Geometry check sheet. Reference: the model listing, model coordinates, mm. Round coordinates to 2 decimals unless told otherwise and drop trailing zeros. Use one line per item in the form item = value.
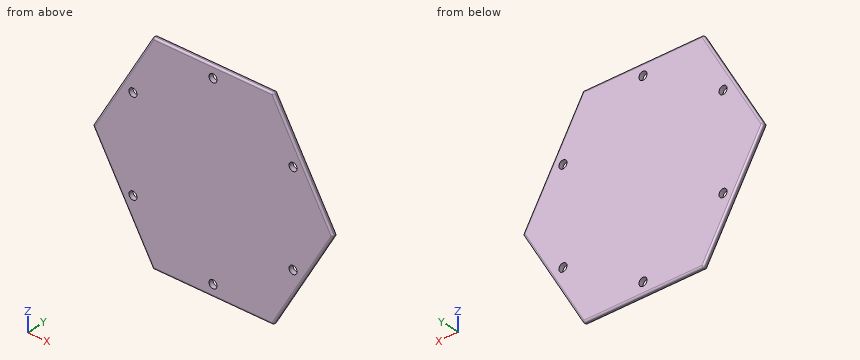
from build123d import *

# Parameters (mm, degrees)
BOSS_EXTRUDE1_DEPTH     = 2
FILLET3_R               = 0.75
CUT_EXTRUDE2_DEPTH      = 69.680097177
CUT_EXTRUDE2_DEPTH_BACK = 35
SKETCH3_R               = 1.75


with BuildPart() as part:
    # Sketch2 → Boss-Extrude1 (new body)
    with BuildSketch(Plane(origin=(0, 0, 0), x_dir=(1, 0, 0), z_dir=(0, 1, 0))):
        Polygon((51.961524227, 0), (25.980762114, 45), (-25.980762114, 45), (-51.961524227, 0), (-25.980762114, -45), (25.980762114, -45), align=None)
    extrude(amount=BOSS_EXTRUDE1_DEPTH)

    # Fillet3
    fillet3_edges = [part.edges().sort_by_distance(p)[0] for p in [
        (25.980762114, 1, 45),
        (-25.980762114, 1, 45),
        (-51.961524227, 1, 0),
        (-25.980762114, 1, -45),
        (25.980762114, 1, -45),
        (51.961524227, 1, 0),
        (0, 2, -45),
        (-38.97114317, 2, -22.5),
        (-38.97114317, 2, 22.5),
        (0, 2, 45),
        (38.97114317, 2, 22.5),
        (0, 0, 45),
        (-38.97114317, 0, 22.5),
        (-38.97114317, 0, -22.5),
        (0, 0, -45),
        (38.97114317, 0, -22.5),
        (38.97114317, 0, 22.5),
        (38.97114317, 2, -22.5),
    ]]
    fillet(fillet3_edges, radius=FILLET3_R)

    # Sketch3 → Cut-Extrude2 (cut, two sides: drawn at the far end of the back side and taken through both)
    with BuildSketch(Plane(origin=(0, 0, 0), x_dir=(1, 0, 0), z_dir=(0, 1, 0)).offset(-CUT_EXTRUDE2_DEPTH_BACK)):
        with Locations(Location((0, 40, 0), (0, 0, 270))):
            Circle(SKETCH3_R)
        with Locations(Location((34.641016151, 20, 0), (0, 0, 270))):
            Circle(SKETCH3_R)
        with Locations(Location((34.641016151, -20, 0), (0, 0, 270))):
            Circle(SKETCH3_R)
        with Locations(Location((0, -40, 0), (0, 0, 270))):
            Circle(SKETCH3_R)
        with Locations(Location((-34.641016151, -20, 0), (0, 0, 270))):
            Circle(SKETCH3_R)
        with Locations(Location((-34.641016151, 20, 0), (0, 0, 270))):
            Circle(SKETCH3_R)
    extrude(amount=CUT_EXTRUDE2_DEPTH + CUT_EXTRUDE2_DEPTH_BACK, mode=Mode.SUBTRACT)


solid = part.part
1. Material ranges on line 1 along Z through (x, y) = (0, 0.9); line 2 along X through (y, z) = (1.55, 20); line 3 along Z through (x, y) = (1.5, 0.35), recorded low to high.
Return value:
line_1 = -45 to -41.75, -38.25 to 38.25, 41.75 to 45
line_2 = -40.34 to -36.39, -32.89 to 32.89, 36.39 to 40.34
line_3 = -44.88 to -40.9, -39.1 to 39.1, 40.9 to 44.88
2. Gauge pin test, flat ends, axial feed: pin 1 (3 mm diameter, centred on x = -34.64, z = 20, fed in from +Y); pin 2 (1 mm diameter, centred on y = 1.5, z = -6, fed in from -X). Record the tip position at first contact, or that the pin passes through.
Return value:
pin_1 = through
pin_2 = -48.77
3. Section check A-A (z = 20). Count the separate pieces of the cut face and the enclosed holes in it, then the cut area to 3 significant figures.
Return value:
separate_pieces = 3
enclosed_holes = 0
area = 147 mm2
